```python
from build123d import *

# Parameters (mm, degrees)
SKETCH_R        = 1.5
PAD_DEPTH       = 6
SKETCH001_R     = 2
POCKET_DEPTH    = 4
CHAMFER_SIZE    = 0.5
CHAMFER001_SIZE = 1


with BuildPart() as part:
    # Sketch → Pad (new body)
    with BuildSketch(Plane.XY):
        Polygon((3.464102, 6), (-3.464102, 6), (-6.928203, 0), (-3.464102, -6), (3.464102, -6), (6.928203, 0), align=None)
        Circle(SKETCH_R, mode=Mode.SUBTRACT)
    extrude(amount=PAD_DEPTH)

    # Sketch001 (on Face9 of Pad) → Pocket (cut)
    with BuildSketch(Plane.XY.offset(6)):
        Circle(SKETCH001_R)
    extrude(amount=-POCKET_DEPTH, mode=Mode.SUBTRACT)

    # Chamfer
    chamfer_edges = [part.edges().sort_by_distance(p)[0] for p in [
        (-2, 0, 6),
    ]]
    chamfer(chamfer_edges, length=CHAMFER_SIZE)

    # Chamfer001
    chamfer001_edges = [part.edges().sort_by_distance(p)[0] for p in [
        (5.196152, -3, 6),
        (5.196152, 3, 6),
        (0, 6, 6),
        (-5.196152, 3, 6),
        (-5.196152, -3, 6),
        (0, -6, 6),
    ]]
    chamfer(chamfer001_edges, length=CHAMFER001_SIZE)


solid = part.part
```
Input: part model. Units: mm. Frame: model coordinates. A direction names the side the tool comes from. Coordinates: 2 decimals unless noted, no trailing zeros. Loops run counter-clockwise (first coordinate to the right, second up) from the corner with the lowest first, then second, coordinate; pieces in that order, holes last. Notation, with made-up numbers: M 5.25,8 L 62.25,8 A37 cw 62.25,46 Z; hole C -22,-12.5 d8. An arc over 180 degrees is marked long. Use a Markdown table: item, result. Add a question column.
1) Section C-C, the plane z = 3.6. Return the cut outline in (x, y).
2) Pin query (flat end, axial travel): P1, Ø3, axis at x = 5.5, z = 4.5, coming from the +Y side. Return the tip coordinate at first contact, or that it passes through.
3) Draft query along X for faces 1 (the flat face through (-4.745, 2.796, 5.493)), 2 (the flat face through (0, 6, 2)), 3 (the cylindrical face through (-1.5, 0.07, 0.99)), 4 (the flat face through (5.22, 2.96, 2.46)). Return one class per face: +X half, -X half, draft (parallel to the pull), parting line (faces both ways), or undercut.
4) Section A-A, the plane z = 1. Return the cut outline in (x, y), plus the area to 3 significant figures.
5) Section B-B, the plane x = 0. Return the cut outline in (y, z).
6) Line query: L1, parallel to Y at x = 0, z = 4.05; L2, parallel to Y at x = 0, z = 0.8; L3, parallel to Z at x = 1.5, y = 1.25. Output: solid intervals per line, ascending. Write a range as from..to.
7) Set-up query: faces 5 (the cylindrical face through (0, -2, 4)), 6 (the flat face through (5.172, -3.042, 2.465)). Return all of +Z, -Z, +X, -X, +Y, -Y with unobstructed straight access to the full face (end or side cutting, diameter ignored); none if empty.
8) Section D-D, the plane y = 3.75. Return the cut outline in (x, z).
Answer below:
| question | item | result |
|---|---|---|
| 1 | outline | M -6.93,0 L -3.46,-6 L 3.46,-6 L 6.93,0 L 3.46,6 L -3.46,6 Z; hole C 0,0 d4 |
| 2 | P1 | y = 5.07 |
| 3 | face 1 | -X half |
| 3 | face 2 | draft |
| 3 | face 3 | undercut |
| 3 | face 4 | +X half |
| 4 | outline | M -6.93,0 L -3.46,-6 L 3.46,-6 L 6.93,0 L 3.46,6 L -3.46,6 Z; hole C 0,0 d3 |
| 4 | area | 118 mm2 |
| 5 | outline | M -6,0 L -1.5,0 L -1.5,2 L -2,2 L -2,5.5 L -2.5,6 L -5,6 L -6,5 Z; M 1.5,0 L 6,0 L 6,5 L 5,6 L 2.5,6 L 2,5.5 L 2,2 L 1.5,2 Z |
| 6 | L1 | -6..-2, 2..6 |
| 6 | L2 | -6..-1.5, 1.5..6 |
| 6 | L3 | 0..2 |
| 7 | face 5 | +Z |
| 7 | face 6 | +Z, -Z, +X, -Y |
| 8 | outline | M -4.76,0 L 4.76,0 L 4.76,5 L 3.61,6 L -3.61,6 L -4.76,5 Z |
